CAD build for the part. Positions are in the model's coordinates, mm. Face numbers are marked on the shaded views. A direction names the side the tool comes from. Coordinates: 2 decimals unless noted, no trailing zeros. Order: outer loops, then holes, each group sorted by start corner. A loop starts at its lowest first (then second) coordinate and runs counter-clockwise, first axis right, second up. Notation, with made-up numbers: (70, -28) - (126, -28) arc R22 cw to (126, 2) - close; hole circle Ø2 at (54.25, 19.25). An arc over 180 degrees is marked (long way). Return JSON: item names as keys, results as strings.
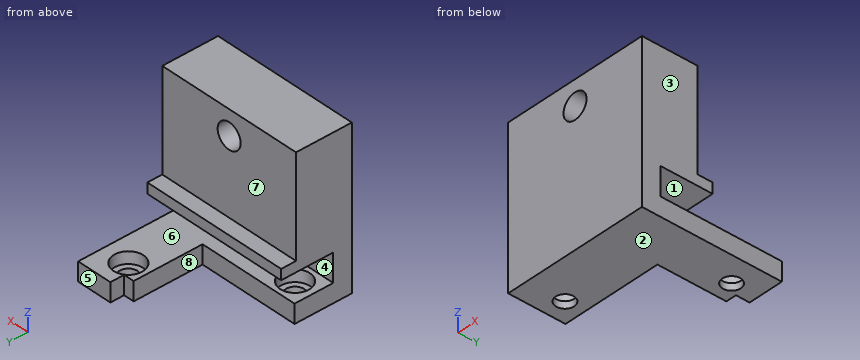
from build123d import *

# Parameters (mm, degrees)
SKETCH2_R           = 1.5748
SKETCH2_W           = 1
SKETCH2_H           = 6.604
BOSS_EXTRUDE1_DEPTH = 3.175
SKETCH3_W           = 25.098
SKETCH3_H           = 3.175
BOSS_EXTRUDE3_DEPTH = 26.67
SKETCH5_R           = 2.54
CUT_EXTRUDE2_DEPTH  = 2
SKETCH6_W           = 25.098
SKETCH6_H           = 18.7325
BOSS_EXTRUDE4_DEPTH = 6.35
SKETCH4_R           = 2.159
CUT_EXTRUDE3_DEPTH  = 39.036194564
SKETCH7_W           = 25.098
SKETCH7_H           = 1.778
BOSS_EXTRUDE5_DEPTH = 2.54


with BuildPart() as part:
    # Sketch2 → Boss-Extrude1 (new body)
    # profile 1 of 2: a face of its own
    with BuildSketch(Plane.XY):
        Polygon((4.395213829, 10.321811953), (4.395213829, 7.827388121), (4.395213829, -1.438404904), (-11.860786171, -1.438404904), (-11.860786171, -8.042404904), (12.237213829, -8.042404904), (12.237213829, 12.658595096), (7.697213829, 12.658595096), (6.188170382, 12.658595096), (6.188170382, 10.321811953), align=None)
        with Locations((-9.320786171, -4.740404904)):
            Circle(SKETCH2_R, mode=Mode.SUBTRACT)
        with Locations((7.697213829, 8.213595096)):
            Circle(SKETCH2_R, mode=Mode.SUBTRACT)
    # profile 2 of 2: a face of its own
    with BuildSketch(Plane.XY):
        with Locations((-12.360786171, -4.740404904)):
            Rectangle(SKETCH2_W, SKETCH2_H)
    extrude(amount=BOSS_EXTRUDE1_DEPTH)

    # Sketch3 → Boss-Extrude3 (add)
    with BuildSketch(Plane(origin=(0, 0, 0), x_dir=(-1, 0, 0), z_dir=(0, 0, -1))):
        with Locations((0.311786171, -9.629904904)):
            Rectangle(SKETCH3_W, SKETCH3_H)
    extrude(amount=-BOSS_EXTRUDE3_DEPTH)

    # Sketch5 → Cut-Extrude2 (cut)
    with BuildSketch(Plane.XY.offset(3.175)):
        with Locations((7.697213829, 8.213595096)):
            Circle(SKETCH5_R)
        with Locations((-9.320786171, -4.740404904)):
            Circle(SKETCH5_R)
    extrude(amount=-CUT_EXTRUDE2_DEPTH, mode=Mode.SUBTRACT)

    # Sketch6 → Boss-Extrude4 (add)
    with BuildSketch(Plane(origin=(0, -8.042404904, 0), x_dir=(1, 0, 0), z_dir=(0, 1, 0))):
        with Locations((-0.311786171, -17.30375)):
            Rectangle(SKETCH6_W, SKETCH6_H)
    extrude(amount=BOSS_EXTRUDE4_DEPTH)

    # Sketch4 → Cut-Extrude3 (cut, through all)
    with BuildSketch(Plane.XZ.offset(11.217404904)):
        with Locations(Location((-0.311786171, 22.479, 0), (0, 0, 270))):
            Circle(SKETCH4_R)
    extrude(amount=-CUT_EXTRUDE3_DEPTH, mode=Mode.SUBTRACT)

    # Sketch7 → Boss-Extrude5 (add)
    with BuildSketch(Plane(origin=(0, -1.692404904, 0), x_dir=(1, 0, 0), z_dir=(0, 1, 0))):
        with Locations((-0.311786171, -8.8265)):
            Rectangle(SKETCH7_W, SKETCH7_H)
    extrude(amount=BOSS_EXTRUDE5_DEPTH)


solid = part.part
Item 1: Mould opens along Z. For the marked faces 1, 2, 3 and 4 say: released by +Z, released by -Z, zero draft, split by the parting line, or undercut.
Findings below:
{"face 1": "undercut", "face 2": "released by -Z", "face 3": "zero draft", "face 4": "undercut"}
Item 2: Wall check: L1, parallel to Z at x = 3.5, y = -4.25 (1 decimal); L2, parallel to Y at x = -5.25, z = 17.25; L3, parallel to X at y = -9, z = 23.5. Give the ranges that are in metal, low to high. Write a range as [from, to].
Findings below:
{"L1": "z = [0, 3.2], [7.9, 26.7]", "L2": "y = [-11.22, -1.69]", "L3": "x = [-12.86, -2.21], [1.59, 12.24]"}
Item 3: Which spindle directions (+Z, -Z, +X, -X, +Y, -Y) get a long thin tool onto all of the face, cutting with end or side? Do the marked faces 5, 6, 7 and 8. Say none if no direction does.
Findings below:
{"face 5": "+Z, -Z, +X, -X, +Y", "face 6": "+X, -X, +Y", "face 7": "+Z, +X, -X, +Y", "face 8": "-Z, -X, +Y"}
Item 4: Band-saw the part on C-C, the plane z = 23.75. List the corners of the cut face in (x, y), then the cut area to 3 significant figures.
Findings below:
{"outline": "(-12.86, -11.22) - (-2.06, -11.22) - (-2.06, -1.69) - (-12.86, -1.69) - close; (1.43, -11.22) - (12.24, -11.22) - (12.24, -1.69) - (1.43, -1.69) - close", "area": "206 mm²"}
Item 5: Band-saw the part on A-A, the plane x = -8.25. List the corners of the cut face in (y, z) (1 decimal), then the cut area to 3 significant figures.
Findings below:
{"outline": "(-11.2, 0) - (-5.9, 0) - (-5.9, 1.2) - (-7, 1.2) - (-7, 3.2) - (-8, 3.2) - (-8, 7.9) - (0.8, 7.9) - (0.8, 9.7) - (-1.7, 9.7) - (-1.7, 26.7) - (-11.2, 26.7) - close; (-3.6, 0) - (-1.4, 0) - (-1.4, 3.2) - (-2.4, 3.2) - (-2.4, 1.2) - (-3.6, 1.2) - close", "area": "217 mm²"}
Item 6: Drop flat-ended pins along their axis: P1, Ø4, axis at x = 7.7, y = 8.21, coming from the -Z side; P2, Ø2, axis at x = 2.5, y = 0, coming from the +Z side; P3, Ø1, axis at x = -6, z = 1.5, coming from the +Y side; P4, Ø3.5, axis at x = -0.31, z = 22.48, coming from the -Y side. Give the stop position or say it passes through.
Findings below:
{"P1": "stops at z = 0", "P2": "stops at z = 9.72", "P3": "stops at y = -1.44", "P4": "passes through"}
Item 7: Band-saw the part on B-B, the plane y = -5.75. List the corners of the cut face in (x, z) (1 decimal).
Findings below:
{"outline": "(-12.9, 0) - (-10.5, 0) - (-10.5, 1.2) - (-11.7, 1.2) - (-11.7, 3.2) - (-12.9, 3.2) - close; (-12.9, 7.9) - (12.2, 7.9) - (12.2, 26.7) - (-12.9, 26.7) - close; (-8.1, 0) - (12.2, 0) - (12.2, 3.2) - (-7, 3.2) - (-7, 1.2) - (-8.1, 1.2) - close; hole circle Ø4.3 at (-0.3, 22.5)"}
Item 8: Band-saw the part on D-D, the plane x = -5. List the corners of the cut face in (y, z) (1 decimal), then the cut area to 3 significant figures.
Findings below:
{"outline": "(-11.2, 0) - (-1.4, 0) - (-1.4, 3.2) - (-8, 3.2) - (-8, 7.9) - (0.8, 7.9) - (0.8, 9.7) - (-1.7, 9.7) - (-1.7, 26.7) - (-11.2, 26.7) - close", "area": "229 mm²"}
